```python
from build123d import *

# Parameters (mm, degrees)
SKETCH006_W     = 609.6
SKETCH006_H     = 63.5
PAD002_DEPTH    = 6.35
SKETCH007_R     = 2.5
POCKET001_DEPTH = 25
SKETCH008_R     = 2.55
POCKET002_DEPTH = 25
SKETCH016_R     = 2.5
POCKET007_DEPTH = 12.701


with BuildPart() as part:
    # Sketch006 → Pad002 (new body, symmetric)
    with BuildSketch(Plane.YZ):
        Rectangle(SKETCH006_W, SKETCH006_H)
    extrude(amount=PAD002_DEPTH, both=True)

    # Sketch007 (on Face4 of Pad002) → Pocket001 (cut)
    with BuildSketch(Plane(origin=(0, -304.8, 0), x_dir=(0, 0, -1), z_dir=(0, -1, 0))):
        Circle(SKETCH007_R)
    pocket001 = extrude(amount=-POCKET001_DEPTH, mode=Mode.SUBTRACT)

    # Mirrored001: Pocket001 across XZ
    add(pocket001.mirror(Plane.XZ), mode=Mode.SUBTRACT)

    # Sketch008 → Pocket002 (cut)
    with BuildSketch(Plane(origin=(0, 0, 31.75), x_dir=(0, -1, 0), z_dir=(0, 0, 1))):
        with Locations((-234.8, 0)):
            Circle(SKETCH008_R)
        with Locations((-78.266667, 0)):
            Circle(SKETCH008_R)
        with Locations((78.266667, 0)):
            Circle(SKETCH008_R)
        with Locations((234.8, 0)):
            Circle(SKETCH008_R)
    pocket002 = extrude(amount=-POCKET002_DEPTH, mode=Mode.SUBTRACT)

    # Mirrored: Pocket002 across XY
    add(pocket002.mirror(Plane.XY), mode=Mode.SUBTRACT)

    # Sketch016 (on Face4 of Mirrored) → Pocket007 (cut, through all)
    with BuildSketch(Plane.YZ.offset(6.35)):
        with Locations((-256.75, 23)):
            Circle(SKETCH016_R)
        with Locations((-256.75, -23)):
            Circle(SKETCH016_R)
        with Locations((-243.75, 23)):
            Circle(SKETCH016_R)
        with Locations((-243.75, -23)):
            Circle(SKETCH016_R)
        with Locations((251.9, 23)):
            Circle(SKETCH016_R)
        with Locations((251.9, -23)):
            Circle(SKETCH016_R)
    extrude(amount=-POCKET007_DEPTH, mode=Mode.SUBTRACT)


with BuildPart() as part_1:
    # Body002 placement: moved
    add(part.part.moved(Location((0, 76, 237))))


solid = part_1.part
```
Could you check a few things on this model? Use its own coordinates, in mm. Give positions to 0.01 mm unless a question says otherwise; leave off trailing zeros. Put each result on its own line as item: value.
(1) Imagine slicing it at A-A on x = 0. State how many separate pieces and enclosed holes the cut face has, plus the area to 3 significant figures.
Computed:
separate pieces: 1
enclosed holes: 6
area: 37,300 mm^2
(2) Please list where these lines run through material, in increasing order: probe 1 along Z at (x, y) = (1, 327.9); probe 2 along Y at (x, z) = (0.5, 222.5); probe 3 along Y at (x, z) = (-0.75, 252). Write a range as [from, to].
Computed:
probe 1: [205.25, 211.5], [216.5, 257.5], [262.5, 268.75]
probe 2: [-228.8, -161.3], [-156.3, -4.77], [0.23, 151.77], [156.77, 308.3], [313.3, 380.8]
probe 3: [-228.8, -161.24], [-156.36, -4.7], [0.17, 151.83], [156.7, 308.36], [313.24, 380.8]
(3) I'm going to push flat-ended pins straight in: pin 1 Ø3 at (x, y) = (0, -2.27) entering from +Z; pin 2 Ø4.5 at (x, y) = (0, 154.27) entering from -Z; pin 3 Ø4.5 at (y, z) = (-180.75, 260) entering from -X; pin 4 Ø4.5 at (x, z) = (0, 237) entering from -Y. Where does each tip first touch, or does it pass through?
Computed:
pin 1: z = 243.75
pin 2: z = 230.25
pin 3: through
pin 4: y = -203.8
